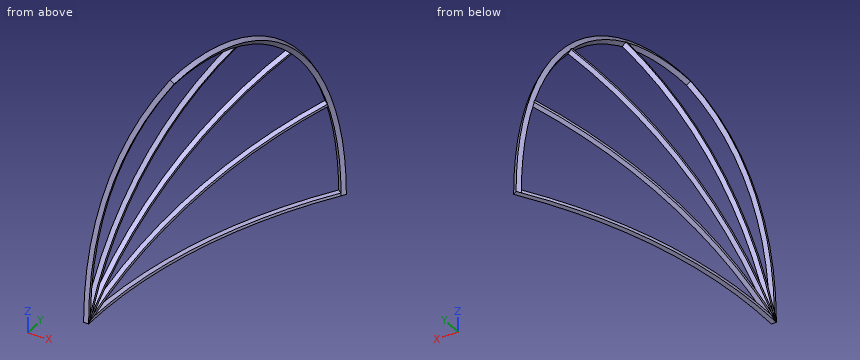
```python
from build123d import *

# Parameters (mm, degrees)
BOSS_EXTRUDE1_DEPTH = 12
CIRPATTERN1_COUNT   = 5
CIRPATTERN1_ANGLE   = 90
CUT_EXTRUDE1_DEPTH  = 357.679347003


with BuildPart() as part:
    # Sketch2 → Boss-Extrude1 (new body)
    with BuildSketch(Plane.XY):
        with BuildLine():
            Line((0, 0), (20, 0))
            ThreePointArc((20, 0), (105.993208992, 584.258082126), (356.679347003, 1118.962485261))
            Line((356.679347003, 1118.962485261), (340, 1129.998761061))
            ThreePointArc((340, 1129.998761061), (86.841356078, 590.020592861), (0, 0))
        make_face()
    boss_extrude1 = extrude(amount=BOSS_EXTRUDE1_DEPTH)

    # CirPattern1: Boss-Extrude1 ×5 about axis
    cirpattern1_axis = Axis((0, 6, 6), (1, 0, 0))
    for i in range(1, CIRPATTERN1_COUNT):
        add(boss_extrude1.rotate(cirpattern1_axis, i * CIRPATTERN1_ANGLE / (CIRPATTERN1_COUNT - 1)))

    # Sketch3 → Cut-Extrude1 (cut, through all)
    with BuildSketch(Plane(origin=(0, 0, 0), x_dir=(0, 0, -1), z_dir=(1, 0, 0))):
        Polygon((0, 0), (0, 11.27415685), (5.748633728, 11.27415685), (5.748633728, -8.438156221), (-12.082999297, -8.438156221), (-12, 0), align=None)
    extrude(amount=CUT_EXTRUDE1_DEPTH, mode=Mode.SUBTRACT)

    # Sweep1: sweep along a path in Sketch5
    with BuildLine(Plane(origin=(0, 0, 0), x_dir=(0, 0, -1), z_dir=(1, 0, 0))) as sweep1_path:
        ThreePointArc((0, 1130), (-799.030662741, 799.030662741), (-1130, 0))
    # Sketch4 → Sweep1 (sweep)
    with BuildSketch(Plane(origin=(0, 0, 0), x_dir=(-1, 0, 0), z_dir=(0, 0, -1))):
        Polygon((-340, 1129.998761061), (-356.679347003, 1118.962485261), (-367.715622804, 1135.641832264), (-351.0362758, 1146.678108065), align=None)
    sweep(path=sweep1_path.line)


solid = part.part
```
Model file for the job. Use its own axes, mm. Coordinates: 2 decimals unless noted, no trailing zeros. Write each loop counter-clockwise with the first axis right and the second up, starting at its lowest first coordinate (ties: lowest second). Pieces come first, ordered by that corner, then holes. Notation, with made-up numbers: (-33, 50) - (-3, 50) arc R22 ccw to (-3, 86) - close; hole circle Ø7 at (-1.75, 19.5). An arc over 180 degrees is marked (long way). Use a Markdown table: item, result. Add a question column.
Item 1: Band-saw the part on B-B, the plane y = 203.5. Give the number of separate pieces and of enclosed holes in the cut face, and give its area (3 significant figures).
Item 2: Drop flat-ended pins along their axis: pin 1 (5 mm diameter, centred on x = 165.5, y = 580.5, fed in from -Z); pin 2 (1 mm diameter, centred on x = 114.5, y = 638.5, fed in from +Z). Give the stop position or say it passes through.
Item 3: Drill centre lines: line 1 along Z through (x, y) = (49.5, 284.5); line 2 along Y through (x, z) = (32, 166); line 3 along Z through (x, y) = (160, 554.5). Where is each one in solid material? Low to high.
Item 4: Band-saw the part on A-A, the plane x = 305. Write the cut outline in (y, z), and give its area (3 significant figures).
A:
| question | item | result |
|---|---|---|
| 1 | separate pieces | 5 |
| 1 | enclosed holes | 0 |
| 1 | area | 1,900 mm² |
| 2 | pin 1 | stops at z = 569.85 |
| 2 | pin 2 | stops at z = 12 |
| 3 | line 1 | z = 276.01 to 292.99 |
| 3 | line 2 | y = 157.51 to 174.49 |
| 3 | line 3 | z = 546.01 to 562.99 |
| 4 | outline | (0, 1036.64) - (12, 1036.64) - (12, 1075.23) - (0, 1075.23) - close; (394.86, 960.48) - (405.95, 955.89) - (420.72, 991.55) - (409.63, 996.14) - close; (730.53, 739.01) - (739.01, 730.53) - (766.3, 757.82) - (757.82, 766.3) - close; (955.89, 405.95) - (960.48, 394.86) - (996.14, 409.63) - (991.55, 420.72) - close; (1036.64, 0) - (1075.23, 0) - (1075.23, 12) - (1036.64, 12) - close |
| 4 | area | 2,320 mm² |
